Part model, mm, in its own coordinate system. Round coordinates to 2 decimals unless told otherwise and drop trailing zeros. Loops run counter-clockwise (first coordinate to the right, second up) from the corner with the lowest first, then second, coordinate; pieces in that order, holes last.
(1) Flat gauge pins, fed straight in: pin 1 (3 mm diameter, centred on x = -1.5, y = -3, fed in from -Z); pin 2 (3 mm diameter, centred on x = 1.5, y = -6, fed in from -Z); pin 3 (2 mm diameter, centred on x = 1, y = 2, fed in from +Z); pin 4 (2 mm diameter, centred on x = -0.5, y = 0.5, fed in from +Z). Where does each tip first touch, or does it go through?
(2) Mould opens along Y. For faces 1 (the face through (2.07, 9.55, -2.12)), 2 (the face through (2.619, 9, -5)), 3 (the face through (0, 6.7, -8.7)) say: +Y half, -Y half, draft (parallel to the pull), parting line (faces both ways), or undercut.
(3) Cut at A-A on y = 0. List the corners of the cut face in (x, z), then the cut area to 3 significant figures.
(4) Probe probe 1 along Y at (x, z) = (-1.85, 0); probe 2 along Z at (x, y) = (1.5, 2.25); probe 3 along Y at (x, z) = (-0.6, 5.75). List the from-to ranges inside material, lowest first.
from build123d import *

# Parameters (mm, degrees)
FILLET1_R    = 2.1
SCALE1_SCALE = 0.22
SCALE2_SCALE = 0.2
SCALE3_SCALE = 3.84


with BuildPart() as part:
    # Sketch1 → Revolve1 (revolve)
    with BuildSketch(Plane.XY, mode=Mode.PRIVATE) as revolve1_sk:
        with BuildLine():
            Line((-15.5, 57.89), (-8.94427191, 57.89))
            ThreePointArc((-8.94427191, 57.89), (0, 61.89), (8.94427191, 57.89))
            Line((8.94427191, 57.89), (15.5, 57.89))
            Line((15.5, 57.89), (15.5, 65))
            Line((15.5, 65), (-15.5, 65))
            Line((-15.5, 65), (-15.5, 57.89))
        make_face()
    revolve(revolve1_sk.sketch.rotate(Axis((-92.395721925, 0, 0), (1, 0, 0)), 90), axis=Axis((-92.395721925, 0, 0), (1, 0, 0)))

    # Fillet1
    fillet1_edges = [part.edges().sort_by_distance(p)[0] for p in [
        (15.5, 0, -65),
        (-15.5, 0, -65),
    ]]
    fillet(fillet1_edges, radius=FILLET1_R)


with BuildPart() as part_1:
    # Scale1: scaled about (0, 0, 0)
    add(part.part.scale(SCALE1_SCALE))


with BuildPart() as part_2:
    # Scale2: scaled about (0, 0, 0)
    add(part_1.part.scale(SCALE2_SCALE))


with BuildPart() as part_3:
    # Scale3: scaled about (0, 0, 0)
    add(part_2.part.scale(SCALE3_SCALE))


solid = part_3.part
Final values:
1. pin 1: stops at z = -10.88
1. pin 2: stops at z = -10.02
1. pin 3: stops at z = 10.94
1. pin 4: stops at z = 10.98
2. face 1: undercut
2. face 2: draft
2. face 3: parting line
3. outline: (-2.62, -10.63) arc R0.35 ccw to (-2.26, -10.98) - (2.26, -10.98) arc R0.35 ccw to (2.62, -10.63) - (2.62, -9.78) - (1.51, -9.78) arc R2.03 cw to (-1.51, -9.78) - (-2.62, -9.78) - close; (-2.62, 9.78) - (-1.51, 9.78) arc R2.03 cw to (1.51, 9.78) - (2.62, 9.78) - (2.62, 10.63) arc R0.35 ccw to (2.26, 10.98) - (-2.26, 10.98) arc R0.35 ccw to (-2.62, 10.63) - close
3. area: 9.65 mm2
4. probe 1: y = -10.98 to -9.78, 9.78 to 10.98
4. probe 2: z = -10.75 to -9.53, 9.53 to 10.75
4. probe 3: y = -9.36 to -8.63, 8.63 to 9.36
